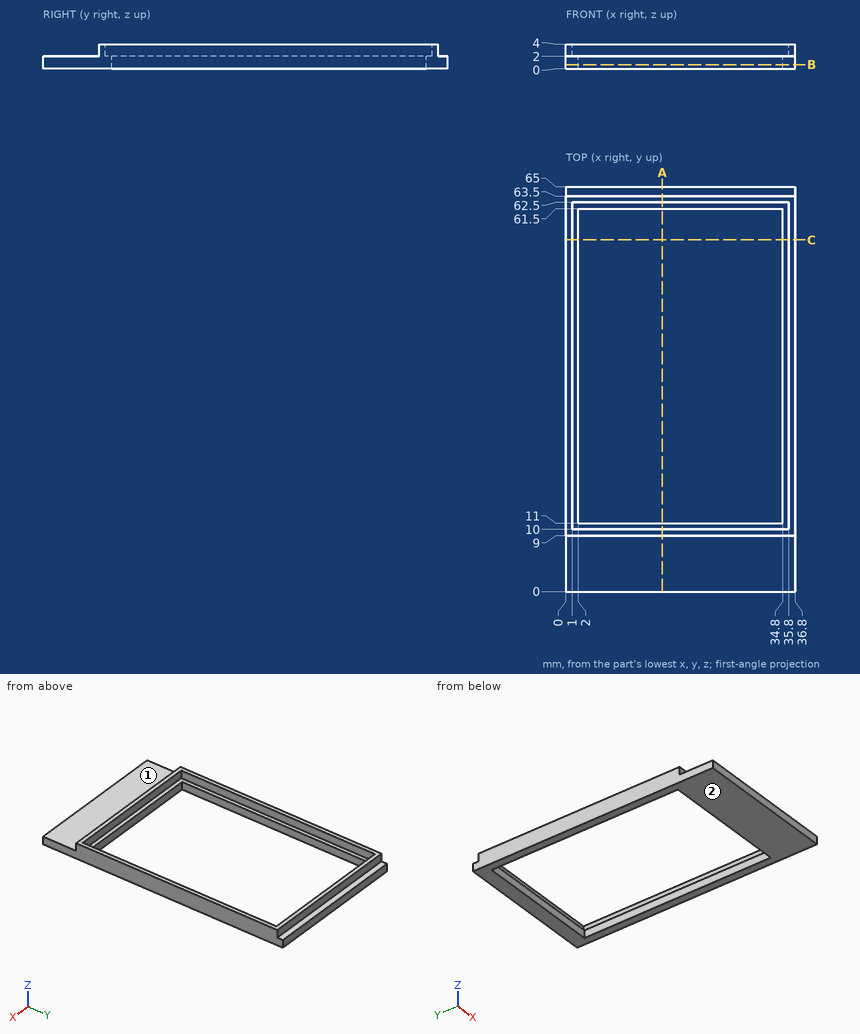
Geometry check sheet. Reference: drawing and pictorial views, mm from the part's lowest x, y, z. A direction names the side the tool comes from. Give positions to 0.01 mm unless a question says otherwise; leave off trailing zeros. Write each loop counter-clockwise with the first axis right and the second up, starting at its lowest first coordinate (ties: lowest second). Pieces come first, ordered by that corner, then holes. Notation, with made-up numbers: (-4, 12) - (4, 12) arc R24 cw to (4, 34) - close; hole circle Ø11 at (-15.5, 47.25). An arc over 180 degrees is marked (long way). Use a Markdown table: item, result.
Q1. Section check B-B, the plane z = 0.7. Enter the section's corners in (x, y).
Computed:
| item | result |
|---|---|
| outline | (0, 0) - (36.8, 0) - (36.8, 65) - (0, 65) - close; hole (2, 11) - (34.8, 11) - (34.8, 61.5) - (2, 61.5) - close |
Q2. Set-up check for the marked faces 1 and 2: record each of +Z, -Z, +X, -X, +Y, -Y from which the full face is reachable in a straight line by a thin tool's end or side.
Computed:
| item | result |
|---|---|
| face 1 | +Z, +X, -X, -Y |
| face 2 | -Z, +X, -X, +Y, -Y |
Q3. Go/stop test with flat-tipped pins: P1, Ø1.2, axis at x = 19, y = 64.5, coming from the +Z side; P2, Ø0.6, axis at x = 25.5, z = 3, coming from the -Y side; P3, Ø6, axis at x = 30.5, y = 20, coming from the +Z side; P4, Ø0.6, axis at x = 27.5, z = 3.5, coming from the +Y side. Record where each tip stops, or that it passes through.
Computed:
| item | result |
|---|---|
| P1 | stops at z = 2 |
| P2 | stops at y = 9 |
| P3 | passes through |
| P4 | stops at y = 63.5 |
Q4. Thickness scan on L1, parallel to X at y = 12.5, z = 0.3; L2, parallel to X at y = 51, z = 3.6; L3, parallel to Y at x = 7, z = 3. Record the ranges inside material, lowest first. Write a range as [from, to].
Computed:
| item | result |
|---|---|
| L1 | x = [0, 2], [34.8, 36.8] |
| L2 | x = [0, 1], [35.8, 36.8] |
| L3 | y = [9, 10], [62.5, 63.5] |
Q5. Section check A-A, the plane x = 15.5. Enter the section's corners in (y, z).
Computed:
| item | result |
|---|---|
| outline | (0, 0) - (11, 0) - (11, 2) - (10, 2) - (10, 4) - (9, 4) - (9, 2) - (0, 2) - close; (61.5, 0) - (65, 0) - (65, 2) - (63.5, 2) - (63.5, 4) - (62.5, 4) - (62.5, 2) - (61.5, 2) - close |
Q6. Section check C-C, the plane y = 56.5. Enter the section's corners in (x, z).
Computed:
| item | result |
|---|---|
| outline | (0, 0) - (2, 0) - (2, 2) - (1, 2) - (1, 4) - (0, 4) - close; (34.8, 0) - (36.8, 0) - (36.8, 4) - (35.8, 4) - (35.8, 2) - (34.8, 2) - close |
